Build history of the part. All positions in model axes, mm. Face numbers are marked on the shaded views. A direction names the side the tool comes from. Round coordinates to 2 decimals unless told otherwise and drop trailing zeros. Write each loop counter-clockwise with the first axis right and the second up, starting at its lowest first coordinate (ties: lowest second). Pieces come first, ordered by that corner, then holes.
1) Saw through at A-A (z = 0). Write the cut outline in (x, y), plus the area to 3 significant figures.
2) Wall check: probe 1 along X at (y, z) = (-1.8, 0); probe 2 along X at (y, z) = (-9.25, 1); probe 3 along Y at (x, z) = (-17, -1.75). Give the ranges that are in metal, low to high.
3) Flat gauge pin, fed straight in: pin 1 (4 mm diameter, centred on x = 15.875, z = 0, fed in from -Y). Where does the tip first touch, or does it go through?
4) Pull direction Z, two halves, no side cores. Call the marked faces 1, 2 and 3: +Z half, -Z half, draft (parallel to the pull), parting line (faces both ways), or undercut.
5) Saw through at B-B (y = -3). Write the cut outline in (x, z) (3 decimals), plus the area to 3 significant figures.
6) Saw through at C-C (y = -10). Write the cut outline in (x, z) (3 decimals), plus the area to 3 significant figures.
7) Saw through at D-D (z = 3.25). Write the cut outline in (x, y).
8) Which spindle directions (+Z, -Z, +X, -X, +Y, -Y) get a long thin tool onto all of the face, cutting with end or side? Do the marked faces 4 and 5. Say none if no direction does.
Autodesk Inventor part; units mm, degrees
ref_plane "YZ Plane" through (0, 0, 0) normal (1, 0, 0) x (0, 1, 0)
ref_plane "XZ Plane" through (0, 0, 0) normal (0, 1, 0) x (-1, 0, 0)
ref_plane "XY Plane" through (0, 0, 0) normal (0, 0, 1) x (1, 0, 0)
sketch "Sketch1" plane through (0, 0, 0) normal (0, 1, 0) x (-1, 0, 0)
  line L0 (25.4, 6.35) -> (-25.4, 6.35)
  line L1 (-25.4, 6.35) -> (-25.4, -6.35)
  line L2 (-25.4, -6.35) -> (25.4, -6.35)
  line L3 (25.4, -6.35) -> (25.4, 6.35)
  line L4 (25.4, 6.35) -> (-25.4, -6.35) construction
  line L5 (-25.4, 6.35) -> (25.4, -6.35) construction
  point P0 (0, 0)
  dimension "d0" = 50.8
  dimension "d1" = 12.7
extrude "Extrusion1" add sketch "Sketch1" against normal blind 12.7
sketch "Sketch3" plane through (-25.4, 0, 6.35) normal (0, 0, 1) x (1, 0, 0)
  line L0 (0, 0) -> (50.8, 0)
  line L1 (0, 0) -> (0, -12.7)
  line L2 (50.8, -12.7) -> (0, -12.7)
  line L3 (50.8, 0) -> (50.8, -12.7)
  circle A0 centre (29.981, 0) radius 6.35
  point P0 (25.4, 0)
extrude "Extrusion2" cut sketch "Sketch3" against normal through all contours A0 L0 | L0 A0
sketch "Sketch4" plane through (0, -12.7, 0) normal (0, -1, 0) x (1, 0, 0)
  line L0 (-25.4, 6.35) -> (-25.4, -6.35) construction
  line L1 (-25.4, 0) -> (25.4, 0) construction
  line L2 (25.4, -6.35) -> (25.4, 6.35) construction
  point P0 (0, 0)
  point P1 (-15.875, 0)
  point P2 (15.875, 0)
  dimension "d6" = 9.525
  dimension "d7" = 9.525
hole "Hole1" at (-15.875, -12.7, 0) at (15.875, -12.7, 0) direction (0, 1, 0) diameter 2.6416 end through all
sketch "Sketch7" plane through (0, -12.7, 0) normal (0, -1, 0) x (1, 0, 0)
  circle A0 centre (-15.875, 0) radius 1.3208
  circle A1 centre (-15.875, 0) radius 2.4257
  circle A2 centre (15.875, 0) radius 1.3208
  circle A3 centre (15.875, 0) radius 2.4257
  point P0 (0, 0)
  dimension "d18" = 4.8514
extrude "Extrusion4" cut sketch "Sketch7" against normal blind 7.1374
properties part number "HoldWormDrive"
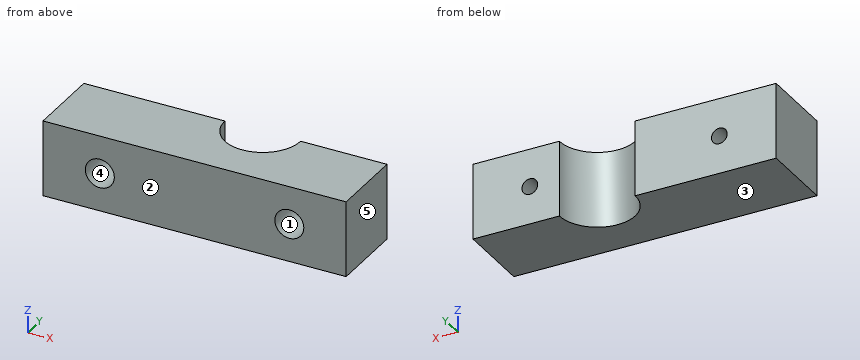
Evaluation:
1. outline: (-25.4, -12.7) - (-18.3, -12.7) - (-18.3, -5.56) - (-17.2, -5.56) - (-17.2, 0) - (-25.4, 0) - close; (-14.55, -5.56) - (-13.45, -5.56) - (-13.45, -12.7) - (13.45, -12.7) - (13.45, -5.56) - (14.55, -5.56) - (14.55, 0) - (10.93, 0) arc R6.35 cw to (-1.77, 0) - (-14.55, 0) - close; (17.2, -5.56) - (18.3, -5.56) - (18.3, -12.7) - (25.4, -12.7) - (25.4, 0) - (17.2, 0) - close
1. area: 483 mm2
2. probe 1: x = -25.4 to -17.2, -14.55 to -1.51, 10.67 to 14.55, 17.2 to 25.4
2. probe 2: x = -25.4 to -18.08, -13.67 to 13.67, 18.08 to 25.4
2. probe 3: y = -5.56 to 0
3. pin 1: stops at y = -5.56
4. face 1: undercut
4. face 2: draft
4. face 3: -Z half
5. outline: (-25.4, -6.35) - (-1.016, -6.35) - (-1.016, 6.35) - (-25.4, 6.35) - close; (10.178, -6.35) - (25.4, -6.35) - (25.4, 6.35) - (10.178, 6.35) - close; hole circle Ø2.642 at (-15.875, 0); hole circle Ø2.642 at (15.875, 0)
5. area: 492 mm2
6. outline: (-25.4, -6.35) - (25.4, -6.35) - (25.4, 6.35) - (-25.4, 6.35) - close; hole circle Ø4.851 at (-15.875, 0); hole circle Ø4.851 at (15.875, 0)
6. area: 608 mm2
7. outline: (-25.4, -12.7) - (25.4, -12.7) - (25.4, 0) - (10.93, 0) arc R6.35 cw to (-1.77, 0) - (-25.4, 0) - close
8. face 4: -Y
8. face 5: +Z, -Z, +X, +Y, -Y
